Can you work these out from the model? Positions are in its coordinate system, mm. Face numbers are marked on the shaded views. A direction names the side the tool comes from. Give positions to 0.01 mm unless a question says otherwise; leave off trailing zeros. Write each loop counter-clockwise with the first axis right and the second up, starting at its lowest first coordinate (ties: lowest second). Pieces come first, ordered by that corner, then holes. Notation, with made-up numbers: (65.5, 76.25) -> (92.5, 76.25) arc R15 ccw to (92.5, 91.25) -> close; hole circle Ø2 at (86, -0.5). An arc over 180 degrees is marked (long way). Answer as CSV lines item,"result". Start each with the question number.
1. If we section it at C-C on y = -73: Write out the boundary of the cut face in (x, z).
2. I'm going to push flat-ended pins straight in: P1, Ø8, axis at x = 4, z = 99.5, coming from the -Y side; P2, Ø0.6, axis at y = -52, z = 241.5, coming from the -X side; P3, Ø10, axis at y = 21, z = 207.5, coming from the -X side; P4, Ø13.5, axis at y = 0, z = 242.32, coming from the -X side. Where does each tip first touch, or does it pass through?
3. If we section it at D-D on z = 38: Write out the boundary of the cut face in (x, y), plus the area to 3 significant figures.
4. On a 3-axis mill with a long thin cutter (end or side, diameter ignored), from which of +Z, -Z, +X, -X, +Y, -Y can I reach the whole of each face in a straight line? I mean the marked faces 1 and 2. Say none if no direction works.
5. I need wall thicknesses on line 1 (Z direction, x = 5, y = 0); line 2 (Z direction, x = -32.5, y = 8.5); line 3 (X direction, y = -35, z = 30). Which ranges of each line are inside material? Lowest first, please. Write a range as [from, to].
6. If we section it at A-A on y = 0: Write out the boundary of the cut face in (x, z).
7. If we section it at B-B on x = 0: Write out the boundary of the cut face in (y, z), plus the area to 3 significant figures.
```python
from build123d import *

# Parameters (mm, degrees)
F0_R     = 45.728615
F1_DEPTH = 203.2
F2_W     = 22.199646
F2_H     = 22.19965
F3_DEPTH = 76.2
F5_DEPTH = 76.2
F7_DEPTH = 25.4


with BuildPart() as f1:
    # F0 (on Top) → F1 (new body)
    with BuildSketch(Plane.XY):
        Circle(F0_R)
    extrude(amount=F1_DEPTH)

    # F2 (on face) → F3 (join)
    with BuildSketch(Plane.XY.offset(203.2)):
        with Locations((-0.98564, 1.738166)):
            Rectangle(F2_W, F2_H)
    extrude(amount=F3_DEPTH)

    # F4 (on face) → F5 (join)
    with BuildSketch(Plane.XZ.offset(9.361659)):
        Polygon((10.114183, 233.951616), (10.114183, 248.648384), (-3.863274, 253.189935), (-12.085463, 241.873063), (-12.085463, 240.726937), (-3.863274, 229.410065), align=None)
    extrude(amount=F5_DEPTH)

    # F6 (on face) → F7 (cut)
    with BuildSketch(Plane.YZ.offset(10.114183)):
        with BuildLine():
            ThreePointArc((-9.361659, 248.648384), (-3.309659, 231.514529), (11.300335, 242.319331))
            ThreePointArc((11.300335, 242.319331), (3.309659, 253.124132), (-9.361659, 248.648384))
        make_face()
    extrude(amount=-F7_DEPTH, mode=Mode.SUBTRACT)


solid = f1.part
```
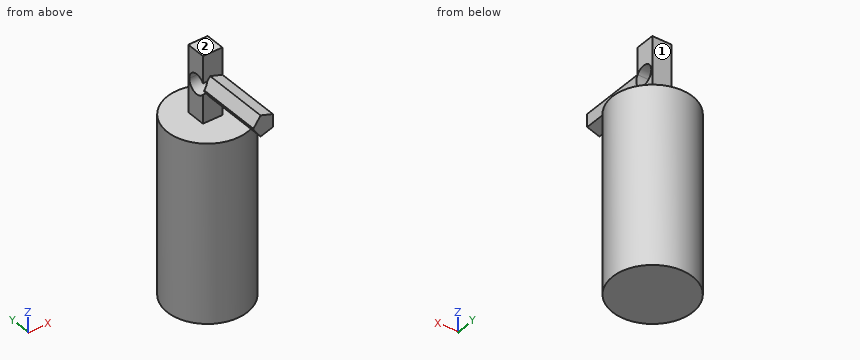
Computed values:
1,outline,"(-12.09, 240.73) -> (-3.86, 229.41) -> (10.11, 233.95) -> (10.11, 248.65) -> (-3.86, 253.19) -> (-12.09, 241.87) -> close"
2,P1,"stops at y = -45.73"
2,P2,"stops at x = -12.09"
2,P3,"stops at x = -41.84"
2,P4,"passes through"
3,outline,"circle Ø91.46 at (0, 0)"
3,area,"6,570 mm2"
4,face 1,"+Z, +X, -X, +Y"
4,face 2,"+Z, +X, -X, +Y, -Y"
5,line 1,"z = [0, 231.02], [253.62, 279.4]"
5,line 2,"z = [0, 203.2]"
5,line 3,"x = [-29.43, 29.43]"
6,outline,"(-45.73, 0) -> (45.73, 0) -> (45.73, 203.2) -> (10.11, 203.2) -> (10.11, 231.02) -> (-12.09, 231.02) -> (-12.09, 203.2) -> (-45.73, 203.2) -> close; (-12.09, 253.62) -> (10.11, 253.62) -> (10.11, 279.4) -> (-12.09, 279.4) -> close"
7,outline,"(-85.56, 230.67) -> (-9.36, 230.67) -> (-9.36, 203.2) -> (-45.73, 203.2) -> (-45.73, 0) -> (45.73, 0) -> (45.73, 203.2) -> (12.84, 203.2) -> (12.84, 279.4) -> (-9.36, 279.4) -> (-9.36, 251.93) -> (-85.56, 251.93) -> close; hole circle Ø22.6 at (0, 242.32)"
7,area,"21,500 mm2"
